Build history of the part. All positions in model axes, mm. A direction names the side the tool comes from. Give positions to 0.01 mm unless a question says otherwise; leave off trailing zeros. Write each loop counter-clockwise with the first axis right and the second up, starting at its lowest first coordinate (ties: lowest second). Pieces come first, ordered by that corner, then holes. Notation, with made-up numbers: M -8,-9.5 L 25,-9.5 A27 cw 25,27.5 Z; hole C -27,71.5 d9. An arc over 180 degrees is marked long. Return JSON: item names as keys, results as strings. Group by question number.
Q1. Band-saw the part on B-B, the plane x = 0. Give the cut face in (y, z), then the cut area to 3 significant figures.
Q2. Band-saw the part on C-C, the plane y = 4.25. Give the cut face in (x, z), then the cut area to 3 significant figures.
Q3. Band-saw the part on D-D, the plane y = 1.75. Give the cut face in (x, z).
Q4. Tool access for faces 3 (the cylindrical face through (4.05, 1.94, -0.9)), 4 (the flat face through (0, 6.3, 0)): list every direction of +Z, -Z, +X, -X, +Y, -Y with a clear straight run to the whole face (end or side of a thin tool).
Q5. Flat gauge pins, fed straight in: pin 1 Ø1 at (y, z) = (5.5, 1) entering from +X; pin 2 Ø1.5 at (x, z) = (9, 8) entering from -Y; pin 3 Ø6.5 at (x, z) = (-2, 1) entering from -Y; pin 4 Ø2 at (x, y) = (2.5, 1.5) entering from -Z. Where does each tip first touch, or does it go through?
Q6. Wall check: probe 1 along Y at (x, z) = (-4.75, 0.25); probe 2 along Y at (x, z) = (-7.25, -4); probe 3 along X at (y, z) = (4, -0.25). Give the ranges that are in metal, low to high.
Q7. Pull direction X, two halves, no side cores. Call faces 1 (the cylindrical face through (-0.49, 4.54, -11.19)), 2 (the flat face through (0, 0, 0)): +X half, -X half, draft (parallel to the pull), parting line (faces both ways), or undercut.
Q8. Band-saw the part on A-A, the plane z = 0. Give the cut face in (x, y).
from build123d import *

# Parameters (mm, degrees)
F2_SIZE = 1


with BuildPart() as f1:
    # F0 (on Right) → F1 (revolve)
    with BuildSketch(Plane.YZ):
        Polygon((0, 0), (6.3, 0), (6.3, 11.2), (3.8, 11.2), (3.8, 6.5), (3, 6.5), (3, 4.15), (0.9, 4.15), (0, 3.95), align=None)
    revolve(axis=Axis((0, 3.15, 0), (0, -1, 0)))

    # F2
    f2_edges = [f1.edges().sort_by_distance(p)[0] for p in [
        (0, 6.3, -11.2),
    ]]
    chamfer(f2_edges, length=F2_SIZE)


solid = f1.part
From the geometry:
{
 "1": {"outline": "M 0,-3.95 L 0.9,-4.15 L 3,-4.15 L 3,-6.5 L 3.8,-6.5 L 3.8,-11.2 L 5.3,-11.2 L 6.3,-10.2 L 6.3,10.2 L 5.3,11.2 L 3.8,11.2 L 3.8,6.5 L 3,6.5 L 3,4.15 L 0.9,4.15 L 0,3.95 Z", "area": "90.1 mm^2"},
 "2": {"outline": "C 0,0 d22.4", "area": "394 mm^2"},
 "3": {"outline": "C 0,0 d8.3"},
 "4": {"face 3": "-Y", "face 4": "+Z, -Z, +X, -X, +Y"},
 "5": {"pin 1": "stops at x = 11.19", "pin 2": "passes through", "pin 3": "stops at y = 0", "pin 4": "stops at z = -3.87"},
 "6": {"probe 1": "y = 3 to 6.3", "probe 2": "y = 3.8 to 6.3", "probe 3": "x = -11.2 to 11.2"},
 "7": {"face 1": "parting line", "face 2": "draft"},
 "8": {"outline": "M -11.2,3.8 L -6.5,3.8 L -6.5,3 L -4.15,3 L -4.15,0.9 L -3.95,0 L 3.95,0 L 4.15,0.9 L 4.15,3 L 6.5,3 L 6.5,3.8 L 11.2,3.8 L 11.2,5.3 L 10.2,6.3 L -10.2,6.3 L -11.2,5.3 Z"}
}
